```python
from build123d import *

# Parameters (mm, degrees)
SKETCH1_W           = 200.025
SKETCH1_H           = 200.025
SKETCH1_R           = 5.08
SKETCH1_W_2         = 27.758924323
SKETCH1_H_2         = 15.850492031
SKETCH1_W_3         = 31.563171913
SKETCH1_H_3         = 7.913427648
BOSS_EXTRUDE1_DEPTH = 6.35
SKETCH2_W           = 200.025
SKETCH2_H           = 200.025
SKETCH2_R           = 5.08
SKETCH2_W_2         = 149.225
SKETCH2_H_2         = 149.225
SKETCH2_W_3         = 27.758924323
SKETCH2_H_3         = 15.874128766
SKETCH2_W_4         = 31.563171913
SKETCH2_H_4         = 7.937064383
BOSS_EXTRUDE2_DEPTH = 6.350254
SKETCH3_R           = 1.00000054
CUT_EXTRUDE1_DEPTH  = 23.622


with BuildPart() as part:
    # Sketch1 → Boss-Extrude1 (new body)
    with BuildSketch(Plane(origin=(0, 0, 0), x_dir=(1, 0, 0), z_dir=(0, 1, 0))):
        with Locations((0, -0.023636735)):
            Rectangle(SKETCH1_W, SKETCH1_H)
        with Locations((-87.3125, 87.288863265)):
            Circle(SKETCH1_R, mode=Mode.SUBTRACT)
        with Locations((87.3125, 87.288863265)):
            Circle(SKETCH1_R, mode=Mode.SUBTRACT)
        with Locations((-87.3125, -87.288863265)):
            Circle(SKETCH1_R, mode=Mode.SUBTRACT)
        with Locations((87.3125, -87.288863265)):
            Circle(SKETCH1_R, mode=Mode.SUBTRACT)
        Polygon((38.5, 54.27), (42.77, 54.27), (42.77, 51.27), (49, 51.27), (51.27, 51.27), (51.27, 49), (51.27, 42.77), (54.27, 42.77), (54.27, 38.5), (54.27, -38.5), (54.27, -42.77), (51.27, -42.77), (51.27, -49), (51.27, -51.293636735), (48.998814015, -51.293636735), (42.77, -51.270990058), (42.77, -54.27), (38.5, -54.27), (-38.5, -54.27), (-42.77, -54.27), (-42.77, -51.270990058), (-48.998814015, -51.293636735), (-51.27, -51.293636735), (-51.27, -49), (-51.27, -42.77), (-54.27, -42.77), (-54.27, -38.5), (-54.27, 38.5), (-54.27, 42.77), (-51.27, 42.77), (-51.27, 49), (-51.27, 51.27), (-49, 51.27), (-42.77, 51.27), (-42.77, 54.27), (-38.5, 54.27), align=None, mode=Mode.SUBTRACT)
        with Locations((-19.766444167, 88.253617249)):
            Rectangle(SKETCH1_W_2, SKETCH1_H_2, mode=Mode.SUBTRACT)
        with Locations((23.505506165, 92.222149441)):
            Rectangle(SKETCH1_W_3, SKETCH1_H_3, mode=Mode.SUBTRACT)
    extrude(amount=BOSS_EXTRUDE1_DEPTH)

    # Sketch2 → Boss-Extrude2 (add)
    with BuildSketch(Plane(origin=(0, 6.35, 0), x_dir=(1, 0, 0), z_dir=(0, 1, 0))):
        Rectangle(SKETCH2_W, SKETCH2_H)
        with Locations((-87.3125, 87.3125)):
            Circle(SKETCH2_R, mode=Mode.SUBTRACT)
        with Locations((87.3125, 87.3125)):
            Circle(SKETCH2_R, mode=Mode.SUBTRACT)
        with Locations((-87.3125, -87.3125)):
            Circle(SKETCH2_R, mode=Mode.SUBTRACT)
        with Locations((87.3125, -87.3125)):
            Circle(SKETCH2_R, mode=Mode.SUBTRACT)
        Rectangle(SKETCH2_W_2, SKETCH2_H_2, mode=Mode.SUBTRACT)
        with Locations((-19.766444167, 88.265435617)):
            Rectangle(SKETCH2_W_3, SKETCH2_H_3, mode=Mode.SUBTRACT)
        with Locations((23.505506165, 92.233967809)):
            Rectangle(SKETCH2_W_4, SKETCH2_H_4, mode=Mode.SUBTRACT)
    extrude(amount=-BOSS_EXTRUDE2_DEPTH)

    # Sketch3 → Cut-Extrude1 (cut)
    with BuildSketch(Plane.XZ):
        with Locations((-33.999932, -66.312542)):
            Circle(SKETCH3_R)
        with Locations((33.999932, -66.312542)):
            Circle(SKETCH3_R)
        with Locations((-66.312542, 33.999932)):
            Circle(SKETCH3_R)
        with Locations((-66.312542, -33.999932)):
            Circle(SKETCH3_R)
        with Locations((33.999932, 66.312542)):
            Circle(SKETCH3_R)
        with Locations((-33.999932, 66.312542)):
            Circle(SKETCH3_R)
        with Locations((66.312542, -33.999932)):
            Circle(SKETCH3_R)
        with Locations((66.312542, 33.999932)):
            Circle(SKETCH3_R)
    extrude(amount=-CUT_EXTRUDE1_DEPTH, mode=Mode.SUBTRACT)


solid = part.part
```
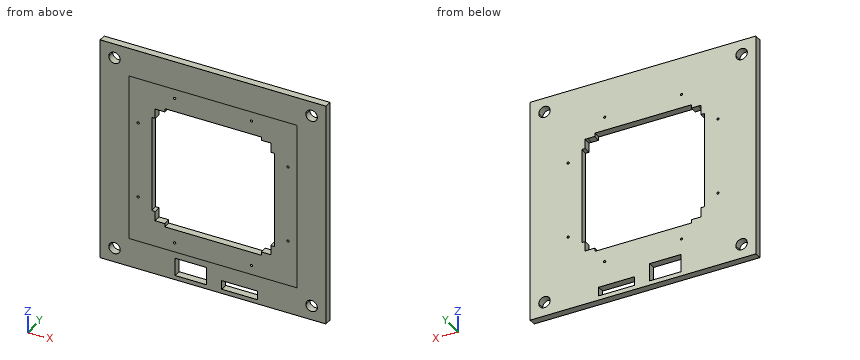
Check sheet for the modelled part. Datum: model origin and axes. Units: mm. Coordinates: 2 decimals unless noted, no trailing zeros. Write item = value, one per line. Start each with the question number.
1) Cross-section at A-A (x = -12). State how many separate pieces and enclosed holes the cut face has, then the cut area to 3 significant figures.
2) Material ranges on L1, parallel to Z at x = -88, y = 5; L2, parallel to Z at x = 30, y = 5.25; L3, parallel to X at y = 3.75, z = -14.5, recorded low to high.
3) Go/stop test with a flat-tipped pin: P1, Ø1.8, axis at x = -66.31, z = 34, coming from the -Y side. Record where the tip stops, or that it passes through.
Ans:
q1.separate_pieces = 3
q1.enclosed_holes = 0
q1.area = 480 mm²
q2.L1 = -100.01 to -92.32, -82.28 to 82.28, 92.32 to 100.04
q2.L2 = -100.01 to -96.18, -88.27 to -54.27, 54.27 to 100.04
q2.L3 = -100.01 to -54.27, 54.27 to 100.01
q3.P1 = through
